```python
from build123d import *

# Parameters (mm, degrees)
F2_DEPTH = 5
F0_R     = 7.5
F0_R_2   = 4
F3_DEPTH = 45
F4_R     = 5
F5_DEPTH = 45


with BuildPart() as f2:
    # F1 (on Top) → F2 (new body)
    with BuildSketch(Plane.XY):
        Polygon((-12.5, -12.5), (0, -12.5), (12.5, -12.5), (12.5, 12.5), (-12.5, 12.5), align=None)
    extrude(amount=F2_DEPTH)

    # F0 (on Top) → F3 (join)
    with BuildSketch(Plane.XY):
        Circle(F0_R)
        Circle(F0_R_2, mode=Mode.SUBTRACT)
    extrude(amount=F3_DEPTH)

    # F4
    f4_edges = [f2.edges().sort_by_distance(p)[0] for p in [
        (12.5, 12.5, 2.5),
        (-12.5, 12.5, 2.5),
        (12.5, -12.5, 2.5),
        (-12.5, -12.5, 2.5),
    ]]
    fillet(f4_edges, radius=F4_R)

    # F0 (on Top) → F5 (cut)
    with BuildSketch(Plane.XY):
        Circle(F0_R_2)
    extrude(amount=F5_DEPTH, mode=Mode.SUBTRACT)


solid = f2.part
```
Check sheet for the modelled part. Datum: model origin and axes. Units: mm. A direction names the side the tool comes from. Coordinates: 2 decimals unless noted, no trailing zeros. Loops run counter-clockwise (first coordinate to the right, second up) from the corner with the lowest first, then second, coordinate; pieces in that order, holes last.
1) Sectioned sample at C-C (z = 4). Record the boundary of the cut face in (x, y), and give its area (3 significant figures).
2) Material ranges on probe 1 along Y at (x, z) = (0, 16); probe 2 along Z at (x, y) = (-9, 7.25); probe 3 along Y at (x, z) = (-3, 32), recorded low to high.
3) Release check for a two-part mould opening along X. For faces 1 (the face through (-0.867, -3.905, 22.185)), 2 (the face through (0, -12.5, 2)), 3 (the face through (-11, -11.07, 2.54)) record: released by +X, released by -X, zero draft, split by the parting line, or undercut.
4) Access from +Z, -Z, +X, -X, +Y, -Y to the whole of each face (thin tool, end or side, straight path). Record for faces 4 (the face through (3, -3, 45)), 5 (the face through (5, 6, 5)).
5) Sectioned sample at D-D (x = -6). Record the boundary of the cut face in (y, z), and give its area (3 significant figures).
6) Gauge pin test, flat ends, axial feed: pin 1 (4 mm diameter, centred on y = -0.5, z = 34, fed in from +X); pin 2 (1 mm diameter, centred on y = 10, z = 4.5, fed in from -X); pin 3 (10 mm diameter, centred on y = -4, z = 12.5, fed in from -X). Record the tip position at first contact, or that the pin passes through.
7) Sectioned sample at A-A (y = 0). Record the boundary of the cut face in (x, z).
Check sheet entries:
1. outline: (-12.5, -7.5) arc R5 ccw to (-7.5, -12.5) - (7.5, -12.5) arc R5 ccw to (12.5, -7.5) - (12.5, 7.5) arc R5 ccw to (7.5, 12.5) - (-7.5, 12.5) arc R5 ccw to (-12.5, 7.5) - close; hole circle Ø8 at (0, 0)
1. area: 553 mm2
2. probe 1: y = -7.5 to -4, 4 to 7.5
2. probe 2: z = 0 to 5
2. probe 3: y = -6.87 to -2.65, 2.65 to 6.87
3. face 1: undercut
3. face 2: zero draft
3. face 3: released by -X
4. face 4: +Z, +X, -X, +Y, -Y
4. face 5: +Z
5. outline: (-12.5, 0) - (12.5, 0) - (12.5, 5) - (4.5, 5) - (4.5, 45) - (-4.5, 45) - (-4.5, 5) - (-12.5, 5) - close
5. area: 485 mm2
6. pin 1: stops at x = 7.5
6. pin 2: stops at x = -12.08
6. pin 3: stops at x = -7.5
7. outline: (-12.5, 0) - (-4, 0) - (-4, 45) - (-7.5, 45) - (-7.5, 5) - (-12.5, 5) - close; (4, 0) - (12.5, 0) - (12.5, 5) - (7.5, 5) - (7.5, 45) - (4, 45) - close
